Input: dimensioned drawing with shaded views. Units: mm. Origin: part minimum x, y, z. A direction names the side the tool comes from. Give positions to 0.01 mm unless a question says otherwise; leave off trailing zeros. Write each loop counter-clockwise with the first axis right and the second up, starting at its lowest first coordinate (ties: lowest second). Pieces come first, ordered by that corner, then holes. Notation, with made-up numbers: M 52.25,-37.75 L 80.25,-37.75 A21 ccw 80.25,-27.75 Z; hole C 73.5,14 d11. An arc over 180 degrees is marked long. Answer as a JSON object with one key per item and string values.
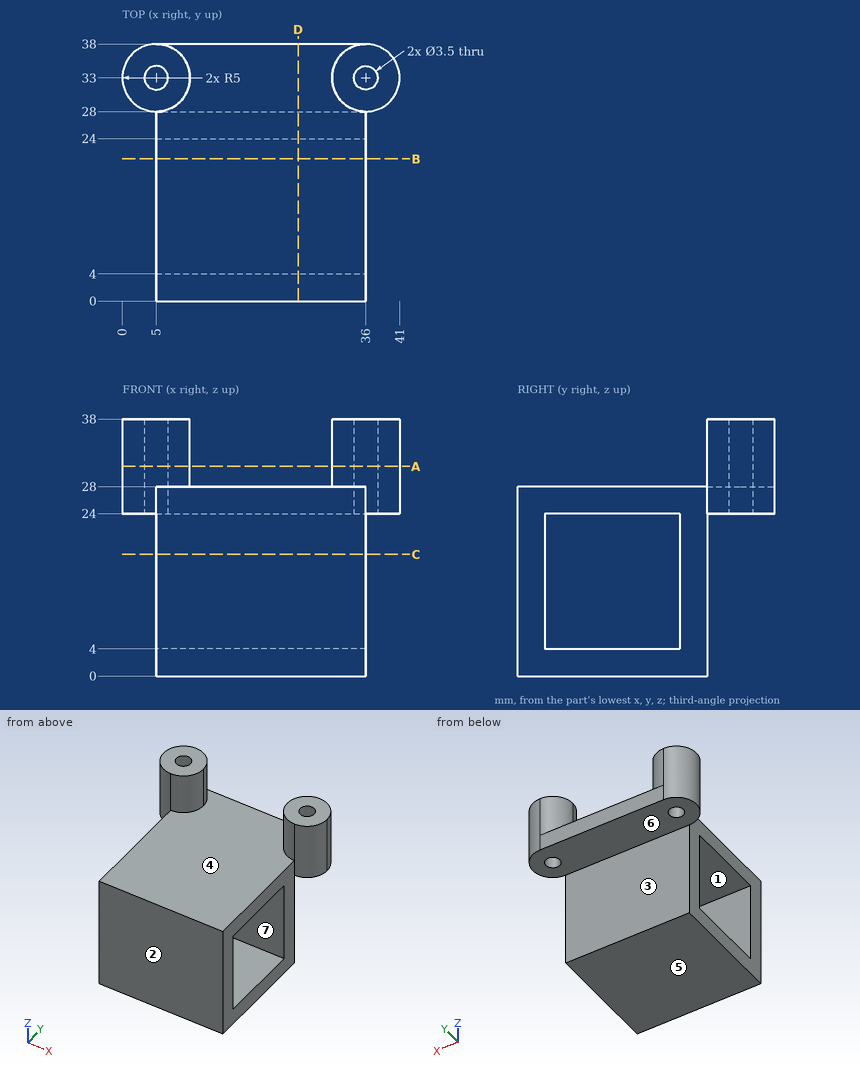
1) Pull-direction query (Y, two-part tool) for the marked faces 1, 2, 3 and 4; classes: pulls with the +Y half, pulls with the -Y half, needs draft (parallel to the pull), parting line crosses it, or undercut.
Geometry check:
{"face 1": "undercut", "face 2": "pulls with the -Y half", "face 3": "pulls with the +Y half", "face 4": "needs draft"}
2) Cut plane A-A on z = 31. Return loops of the section in (x, y).
Geometry check:
{"outline": "C 5,33 d10; C 36,33 d10; hole C 5,33 d3.5; hole C 36,33 d3.5"}
3) Cut plane B-B on y = 21. Return loops of the section in (x, z), and give its area (3 significant figures).
Geometry check:
{"outline": "M 5,0 L 36,0 L 36,4 L 5,4 Z; M 5,24 L 36,24 L 36,28 L 5,28 Z", "area": "248 mm2"}
4) Line query: line 1 (Y direction, x = 15, z = 22); line 2 (Z direction, x = 3.5, y = 29.5); line 3 (Y direction, x = 5, z = 30). Output: solid intervals per line, ascending. Write a range as from..to.
Geometry check:
{"line 1": "y = 0..4, 24..28", "line 2": "z = 24..38", "line 3": "y = 28..31.25, 34.75..38"}
5) Set-up query: the marked faces 5, 6 and 7. Return all of +Z, -Z, +X, -X, +Y, -Y with unobstructed straight access to the full face (end or side cutting, diameter ignored); none if empty.
Geometry check:
{"face 5": "-Z, +X, -X, +Y, -Y", "face 6": "-Z, +X, -X, +Y", "face 7": "+X, -X"}
6) Contact query for flat-ended pins moving along their axis: P1, Ø9.5, axis at x = 19, y = 15.5, coming from the +Z side; P2, Ø16, axis at x = 17.5, y = 13, coming from the -Z side; P3, Ø22.5, axis at y = 15.5, z = 15.5, coming from the -X side; P4, Ø8, axis at y = 10, z = 12.5, coming from the +X side. Output: stop coordinate, or through.
Geometry check:
{"P1": "stops at z = 28", "P2": "stops at z = 0", "P3": "stops at x = 5", "P4": "passes through"}
7) Cut plane D-D on x = 26. Return loops of the section in (y, z), and give its area (3 significant figures).
Geometry check:
{"outline": "M 0,0 L 28,0 L 28,24 L 38,24 L 38,28 L 0,28 Z; hole M 4,4 L 24,4 L 24,24 L 4,24 Z", "area": "424 mm2"}
